Input: dimensioned drawing with shaded views. Units: mm. Origin: part minimum x, y, z. A direction names the side the tool comes from. Round coordinates to 2 decimals unless told otherwise and drop trailing zeros. Loops run counter-clockwise (first coordinate to the right, second up) from the corner with the lowest first, then second, coordinate; pieces in that order, holes last. Notation, with made-up numbers: (-21.5, 18.5) - (17.5, 18.5) arc R35 ccw to (17.5, 53.5) - close; hole circle Ø9 at (5, 81.5). An arc over 180 degrees is marked (long way). One line per question, with ' | ' between items.
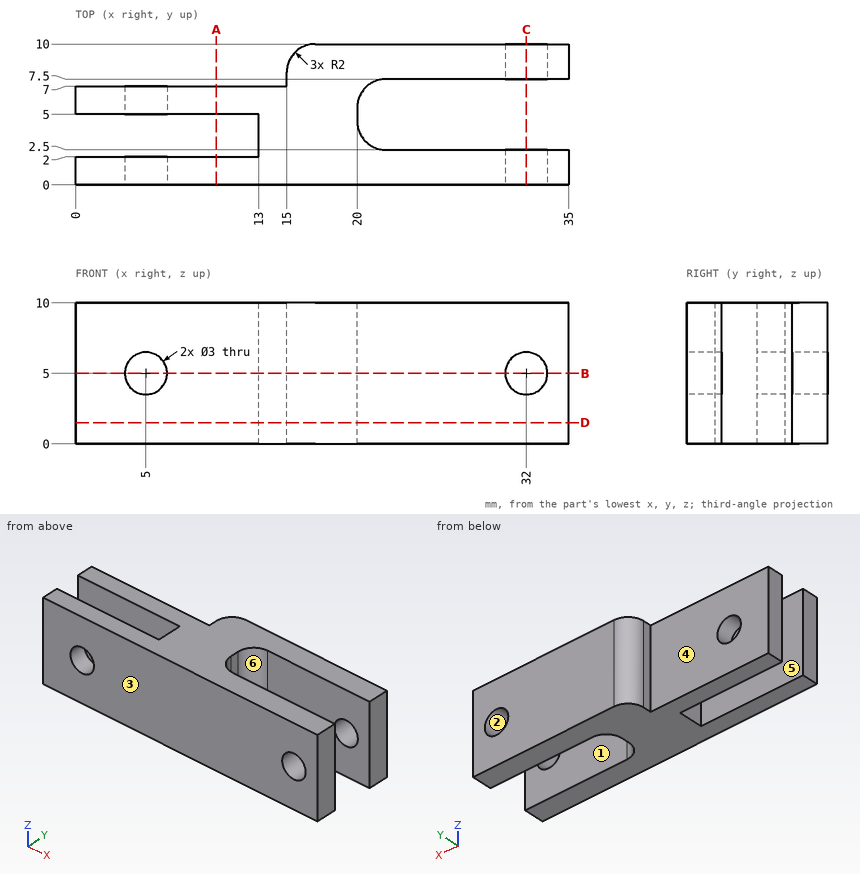
1. Material intervals for probe 1 along X at (y, z) = (1.2, 5); probe 2 along Z at (x, y) = (32, 1.15); probe 3 along Y at (x, z) = (25.5, 6.75), sorted ascending.
Worked out:
probe 1: x = 0 to 3.5, 6.5 to 30.5, 33.5 to 35 | probe 2: z = 0 to 3.5, 6.5 to 10 | probe 3: y = 0 to 2.5, 7.5 to 10
2. Section query B-B, the plane z = 5. Give the number of separate pieces and of enclosed holes in the cut face, plus the area to 3 significant figures.
Worked out:
separate pieces: 5 | enclosed holes: 0 | area: 165 mm2
3. Mould query, pull axis Y, two halves, no side actions, for the marked faces 1, 2 and 3. Classes: released by +Y, released by -Y, zero draft, split by the parting line, or undercut.
Worked out:
face 1: undercut | face 2: zero draft | face 3: released by -Y
4. Section query A-A, the plane x = 10. Return loops of the section in (y, z), plus the area to 3 significant figures.
Worked out:
outline: (0, 0) - (2, 0) - (2, 10) - (0, 10) - close; (5, 0) - (7, 0) - (7, 10) - (5, 10) - close | area: 40.0 mm2
5. Contact query for flat-ended pins moving along their axis: P1, Ø1, axis at x = 12, z = 7, coming from the +Y side; P2, Ø2.5, axis at y = 3, z = 6, coming from the -X side; P3, Ø0.8, axis at y = 5, z = 3, coming from the +X side. Output: stop coordinate, or through.
Worked out:
P1: stops at y = 7 | P2: stops at x = 0 | P3: stops at x = 20
6. Access query for the marked faces 4, 5 and 6. Directions: +Z, -Z, +X, -X, +Y, -Y. A direction counts if a zero-diameter tool reaches every point of the face in a straight line with its end or side. Return the directions, or none.
Worked out:
face 4: +Z, -Z, -X, +Y | face 5: +Z, -Z, -X | face 6: +Z, -Z, +X
7. Section query C-C, the plane x = 32. Return loops of the section in (y, z), plus the area to 3 significant figures.
Worked out:
outline: (0, 0) - (2.5, 0) - (2.5, 3.5) - (0, 3.5) - close; (0, 6.5) - (2.5, 6.5) - (2.5, 10) - (0, 10) - close; (7.5, 0) - (10, 0) - (10, 3.5) - (7.5, 3.5) - close; (7.5, 6.5) - (10, 6.5) - (10, 10) - (7.5, 10) - close | area: 35.0 mm2
8. Section query D-D, the plane z = 1.5. Return loops of the section in (x, y), plus the area to 3 significant figures.
Worked out:
outline: (0, 0) - (35, 0) - (35, 2.5) - (22, 2.5) arc R2 cw to (20, 4.5) - (20, 5.5) arc R2 cw to (22, 7.5) - (35, 7.5) - (35, 10) - (17, 10) arc R2 ccw to (15, 8) - (15, 7) - (0, 7) - (0, 5) - (13, 5) - (13, 2) - (0, 2) - close | area: 192 mm2
